Autodesk Inventor part; units mm, degrees
ref_plane "YZ Plane" through (0, 0, 0) normal (1, 0, 0) x (0, 1, 0)
ref_plane "XZ Plane" through (0, 0, 0) normal (0, 1, 0) x (-1, 0, 0)
ref_plane "XY Plane" through (0, 0, 0) normal (0, 0, 1) x (1, 0, 0)
sketch "Sketch1" plane through (0, 0, 0) normal (1, 0, 0) x (0, 1, 0)
  line L0 (0, 0) -> (10.7, 0)
  line L1 (10.7, 0) -> (10.7, -31.5)
  line L2 (10.7, -31.5) -> (0, -31.5)
  line L3 (0, -31.5) -> (0, 0)
  line L4 (0, 0) -> (-20, 0)
  line L5 (-20, 0) -> (-20, -11.5)
  line L6 (-20, -11.5) -> (0, -11.5)
  line L7 (0, -11.5) -> (0, 0)
  line L8 (-20, -6.8471) -> (-12.0113, -11.5)
  dimension "d0" = 10.7
  dimension "d1" = 11.5
  dimension "d2" = 20
  dimension "d4" = 20
extrude "Extrusion1" add sketch "Sketch1" along normal blind 100 contours L0 L1 L2 L3 | L3 L6 L8 L5 L4
sketch "Sketch2" plane through (0, 0, 0) normal (-1, 0, 0) x (0, 0, 1)
  line L0 (0, -20) -> (-6.8471, -20)
  line L1 (0, 10.7) -> (0, -20)
  line L2 (-31.5, 10.7) -> (0, 10.7)
  line L3 (-31.5, 0) -> (-31.5, 10.7)
  line L4 (-11.5, 0) -> (-31.5, 0)
  line L5 (-11.5, -12.0113) -> (-11.5, 0)
  line L6 (-6.8471, -20) -> (-11.5, -12.0113)
  line L7 (-31.5, 10.7) -> (0, 10.7)
  line L8 (0, 10.7) -> (0, 9)
  line L9 (0, 9) -> (-31.5, 9)
  line L10 (-31.5, 9) -> (-31.5, 10.7)
  point P0 (0, 0)
  dimension "d7" = 1.7
extrude "Extrusion2" cut sketch "Sketch2" against normal blind 40 contours L9 L3 L2 L1
sketch "Sketch3" plane through (0, 0, -31.5) normal (0, -1, 0) x (1, 0, 0)
  line L0 (0, 20) -> (0, 0)
  line L1 (0, 0) -> (100, 0)
  line L2 (100, 20) -> (100, 0)
  line L3 (0, 20) -> (100, 20)
  circle A0 centre (80, 8) radius 1.65
  line L4 (50, 0) -> (50, 9.65)
  circle A1 centre (20, 8) radius 1.65
  point P0 (0, 31.5)
  dimension "d10" = 3.3
  dimension "d11" = 8
  dimension "d12" = 20
extrude "Extrusion3" cut sketch "Sketch3" against normal blind 40 contours A0 | A1
ref_plane "Work Plane1" through (0, 3, -31.5) normal (0, -1, 0) x (1, 0, 0)
sketch "Sketch4" plane through (0, 3, -31.5) normal (0, -1, 0) x (1, 0, 0)
  circle A0 centre (80, 8) radius 1.65
  circle A1 centre (20, 8) radius 1.65
  line L0 (80, 4.6514) -> (77.1, 6.3257)
  line L1 (77.1, 6.3257) -> (77.1, 9.6743)
  line L2 (77.1, 9.6743) -> (80, 11.3486)
  line L3 (80, 11.3486) -> (82.9, 9.6743)
  line L4 (82.9, 9.6743) -> (82.9, 6.3257)
  line L5 (82.9, 6.3257) -> (80, 4.6514)
  line L6 (82.9, 6.3257) -> (82.9, 0)
  line L7 (40, 0) -> (100, 0)
  line L8 (77.1, 6.3257) -> (77.1, 0)
  line L9 (82.9, 0) -> (77.1, 0)
  line L10 (0, 0) -> (100, 0)
  line L11 (50, 0) -> (50, 11.3486)
  circle A2 centre (20, 8) radius 1.65
  line L12 (20, 4.6514) -> (22.9, 6.3257)
  line L13 (22.9, 6.3257) -> (22.9, 9.6743)
  line L14 (22.9, 9.6743) -> (20, 11.3486)
  line L15 (20, 11.3486) -> (17.1, 9.6743)
  line L16 (17.1, 9.6743) -> (17.1, 6.3257)
  line L17 (17.1, 6.3257) -> (20, 4.6514)
  line L18 (17.1, 6.3257) -> (17.1, 0)
  line L19 (22.9, 6.3257) -> (22.9, 0)
  line L20 (17.1, 0) -> (22.9, 0)
  point P0 (0, 31.5)
  point P1 (17.1, 0)
  point P2 (22.9, 0)
  dimension "d16" = 5.8
extrude "Extrusion4" cut sketch "Sketch4" against normal blind 3 contours A0 | L5 L6 L7 L8 L0 | L0 L1 L2 L3 L4 L5 | L10 L18 L17 L12 L19 | L12 L17 L16 L15 L14 L13
properties part number "ESQUINA_RECTA_SUPERIOR" material "Steel, Mild, Welded"
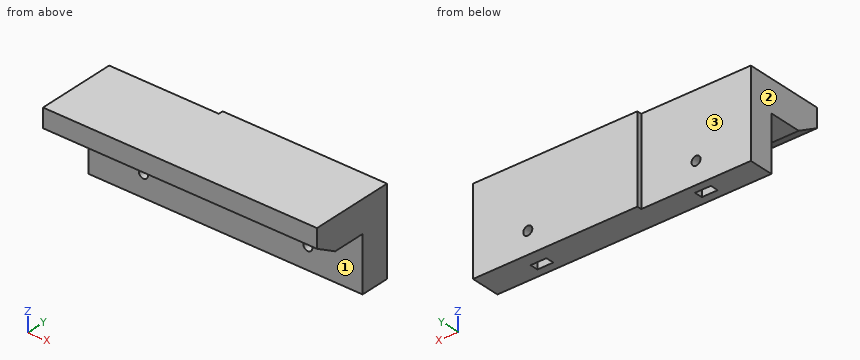
Part model, mm, in its own coordinate system. Face numbers are marked on the shaded views. A direction names the side the tool comes from. Coordinates: 2 decimals unless noted, no trailing zeros. Order: outer loops, then holes, each group sorted by start corner. A loop starts at its lowest first (then second) coordinate and runs counter-clockwise, first axis right, second up.
(1) Slice it at B-B, the plane x = 53.5. Write the cut outline in (y, z), and give its area (3 significant figures).
Check sheet entries:
outline: (-20, -6.85) - (-12.01, -11.5) - (0, -11.5) - (0, -31.5) - (10.7, -31.5) - (10.7, 0) - (-20, 0) - close
area: 548 mm2
(2) Slice it at A-A, the plane z = -23.5. State how many separate pieces and enclosed holes the cut face has, and give its area (3 significant figures).
Check sheet entries:
separate pieces: 3
enclosed holes: 0
area: 922 mm2
(3) Slice it at D-D, the plane y = -10.5. Write the cut outline in (x, z).
Check sheet entries:
outline: (0, -11.5) - (100, -11.5) - (100, 0) - (0, 0) - close
(4) Pin check, flat tips, straight feed: pin 1 Ø4 at (x, z) = (24.5, -11) entering from +Y; pin 2 Ø4.5 at (x, z) = (19.5, -26.5) entering from -Y; pin 3 Ø4 at (x, y) = (29, -7.5) entering from -Z. Stop position of each tip, or through.
Check sheet entries:
pin 1: stops at y = 9
pin 2: stops at y = 0
pin 3: stops at z = -11.5
(5) Tool access for the marked faces 1, 2 and 3: list every direction of +Z, -Z, +X, -X, +Y, -Y with a clear straight run to the whole face (end or side of a thin tool).
Check sheet entries:
face 1: -Z, +X, -X, -Y
face 2: +Z, -Z, -X, +Y, -Y
face 3: +Z, -Z, -X, +Y
(6) Probe L1, parallel to Z at x = 80, y = 1; L2, parallel to Y at x = 79, z = -22; L3, parallel to Y at x = 60, z = -26. List the from-to ranges inside material, lowest first.
Check sheet entries:
L1: z = -31.5 to -25.15, -21.85 to 0
L2: y = 0 to 3, 6 to 10.7
L3: y = 0 to 10.7
(7) Slice it at C-C, the plane z = -17. Write the cut outline in (x, y).
Check sheet entries:
outline: (0, 0) - (100, 0) - (100, 10.7) - (40, 10.7) - (40, 9) - (0, 9) - close
